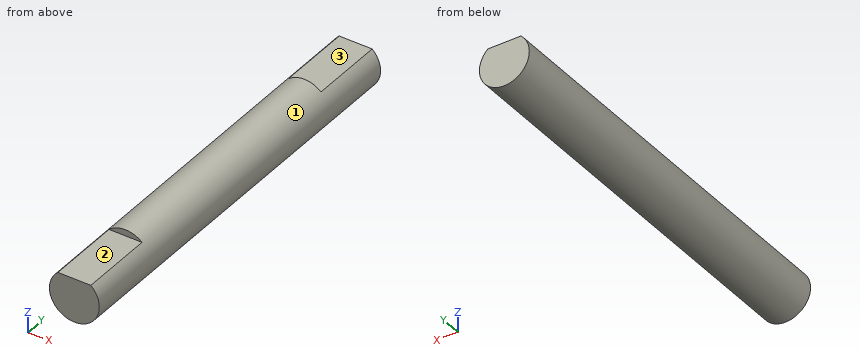
```python
from build123d import *

# Parameters (mm, degrees)
SKETCH2_R               = 4
BOSS_EXTRUDE2_DEPTH     = 66
CUT_EXTRUDE1_START      = -12
CUT_EXTRUDE1_DEPTH      = 12
CUT_EXTRUDE3_DEPTH      = 67.241980647
CUT_EXTRUDE3_DEPTH_BACK = 12


with BuildPart() as part:
    # Sketch2 → Boss-Extrude2 (new body)
    with BuildSketch(Plane(origin=(0, 0, 0), x_dir=(1, 0, 0), z_dir=(0, 1, 0))):
        with Locations(Location((0, 0, 0), (0, 0, 270))):
            Circle(SKETCH2_R)
    extrude(amount=BOSS_EXTRUDE2_DEPTH)

    # Sketch3 → Cut-Extrude1 (cut)
    with BuildSketch(Plane(origin=(0, 66, 0), x_dir=(1, 0, 0), z_dir=(0, 1, 0)).offset(CUT_EXTRUDE1_START)):
        with BuildLine():
            Line((-2.645751311, -3), (2.645751311, -3))
            ThreePointArc((2.645751311, -3), (0, -4), (-2.645751311, -3))
        make_face()
    extrude(amount=CUT_EXTRUDE1_DEPTH, mode=Mode.SUBTRACT)

    # Sketch4 → Cut-Extrude3 (cut, two sides: drawn at the far end of the back side and taken through both)
    with BuildSketch(Plane.XZ.offset(-CUT_EXTRUDE3_DEPTH_BACK)):
        with BuildLine():
            ThreePointArc((2.645751311, 3), (0, 4), (-2.645751311, 3))
            Line((-2.645751311, 3), (2.645751311, 3))
        make_face()
    extrude(amount=CUT_EXTRUDE3_DEPTH + CUT_EXTRUDE3_DEPTH_BACK, mode=Mode.SUBTRACT)


solid = part.part
```
Verification items for the finished model (mm, model axes). Face numbers are marked on the shaded views. A direction names the side the tool comes from. Round coordinates to 2 decimals unless told otherwise and drop trailing zeros. Write each loop counter-clockwise with the first axis right and the second up, starting at its lowest first coordinate (ties: lowest second). Pieces come first, ordered by that corner, then holes. Notation, with made-up numbers: (81.25, 55.25) - (102.25, 55.25) arc R16 cw to (102.25, 84.25) - close; hole circle Ø11 at (41, 34). An arc over 180 degrees is marked (long way). Answer as a JSON object with one key per item and string values. Group by question number.
Q1. Thickness scan on line 1 (X direction, y = 38.5, z = -0.25); line 2 (Y direction, x = -1, z = 3.75); line 3 (X direction, y = 45.5, z = -3.25). Record the ranges inside material, lowest first.
Q2. Go/stop test with flat-tipped pins: pin 1 Ø0.5 at (x, z) = (1, 3.5) entering from +Y; pin 2 Ø2.5 at (x, y) = (1, 8.5) entering from +Z. Record where each tip stops, or that it passes through.
Q3. Section check B-B, the plane y = 58. Enter the section's corners in (x, z).
Q4. Section check A-A, the plane x = 0. Enter the section's corners in (y, z), plus the area to 3 significant figures.
Q5. Tool access check on the marked faces 1, 2 and 3. Record the directions out of +Z, -Z, +X, -X, +Y, -Y that give a thin tool (end or side, any length) a straight path to the whole face; none if there is none.
Q6. Section check C-C, the plane z = 1.5. Enter the section's corners in (x, y).
Q7. Section check D-D, the plane y = 26. Enter the section's corners in (x, z).
Found:
{
 "1": {"line 1": "x = -3.99 to 3.99", "line 2": "y = 12 to 54", "line 3": "x = -2.33 to 2.33"},
 "2": {"pin 1": "stops at y = 54", "pin 2": "stops at z = 3"},
 "3": {"outline": "(-2.65, 3) arc R4 ccw (long way) to (2.65, 3) - close"},
 "4": {"outline": "(0, -4) - (66, -4) - (66, 3) - (54, 3) - (54, 4) - (12, 4) - (12, 3) - (0, 3) - close", "area": "504 mm^2"},
 "5": {"face 1": "+Y, -Y", "face 2": "+Z, +X, -X, -Y", "face 3": "+Z, +X, -X, +Y"},
 "6": {"outline": "(-3.71, 0) - (3.71, 0) - (3.71, 66) - (-3.71, 66) - close"},
 "7": {"outline": "circle Ø8 at (0, 0)"}
}
